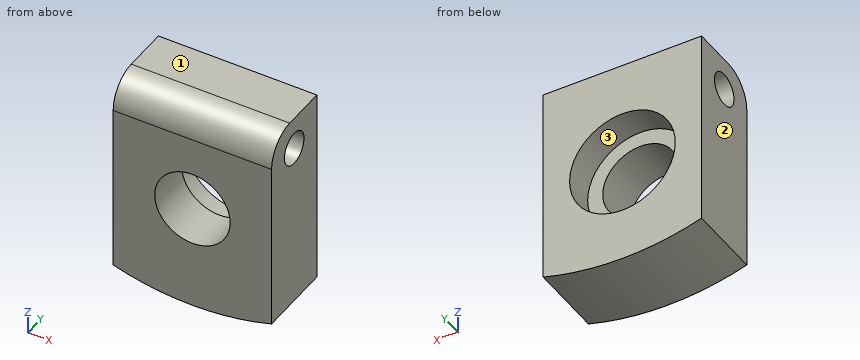
```python
from build123d import *

# Parameters (mm, degrees)
F1_DEPTH       = 30
F3_D           = 30
F3_CBORE_D     = 42
F3_CBORE_DEPTH = 12
F5_R           = 12
F6_D           = 13


with BuildPart() as f1:
    # F0 (on Front) → F1 (new body)
    with BuildSketch(Plane.XZ):
        with BuildLine():
            Line((31.5, 52.105192), (-31.5, 52.105192))
            Line((-31.5, 52.105192), (-31.5, -27.19897))
            ThreePointArc((-31.5, -27.19897), (0, -31.894808), (31.5, -27.19897))
            Line((31.5, -27.19897), (31.5, 52.105192))
        make_face()
    extrude(amount=F1_DEPTH)

    # F3 (through all)
    with Locations(Plane(origin=(0, 0, 0), x_dir=(-1, 0, 0), z_dir=(0, 1, 0))):
        with Locations((0, 10.105192)):
            CounterBoreHole(F3_D / 2, F3_CBORE_D / 2, F3_CBORE_DEPTH)

    # F5
    f5_edges = [f1.edges().sort_by_distance(p)[0] for p in [
        (0, -30, 52.105192),
    ]]
    fillet(f5_edges, radius=F5_R)

    # F6 (through all)
    with Locations(Plane.YZ.offset(31.5)):
        with Locations((-15, 39.105192)):
            Hole(F6_D / 2)


solid = f1.part
```
Check sheet for the modelled part. Datum: model origin and axes. Units: mm. Face numbers are marked on the shaded views. Round coordinates to 2 decimals unless told otherwise and drop trailing zeros. Loops run counter-clockwise (first coordinate to the right, second up) from the corner with the lowest first, then second, coordinate; pieces in that order, holes last. Notation, with made-up numbers: (6.5, 51.25) - (25.5, 51.25) arc R24 ccw to (25.5, 67.25) - close; hole circle Ø5 at (9, 83.25). An arc over 180 degrees is marked (long way). Answer as a JSON object with one key per item and string values. Group by question number.
Q1. Sectioned sample at B-B, the plane x = 0. Enter the section's corners in (y, z), plus the area to 3 significant figures.
Q2. Sectioned sample at D-D, the plane y = -24.25. Enter the section's corners in (x, z).
Q3. Scan lines: line 1 along Z through (x, y) = (0, -7); line 2 along Z through (x, y) = (-7, -12.25); line 3 along Z through (x, y) = (17.5, -9.75). Record each from-to range of solid material in increasing order. Write a range as [from, to].
Q4. Mould release check, pull along Z, two halves, no side actions. Record for the marked faces 1, 2 and 3: released by +Z, released by -Z, zero draft, split by the parting line, or undercut.
Q5. Sectioned sample at C-C, the plane z = -0.5. Enter the section's corners in (x, y).
Q6. Sectioned sample at A-A, the plane y = -15. Enter the section's corners in (x, z), plus the area to 3 significant figures.
Q7. Gauge pin test, flat end, axial feed: P1, Ø8, axis at x = 1, y = -15.5, coming from the -Z side. Record the tip position at first contact, or that the pin passes through.
Solution:
{
 "1": {"outline": "(-30, -31.89) - (0, -31.89) - (0, -10.89) - (-12, -10.89) - (-12, -4.89) - (-30, -4.89) - close; (-30, 25.11) - (-12, 25.11) - (-12, 31.11) - (0, 31.11) - (0, 52.11) - (-18, 52.11) arc R12 ccw to (-30, 40.11) - close; hole circle Ø13 at (-15, 39.11)", "area": "1,310 mm²"},
 "2": {"outline": "(-31.5, -27.2) arc R108 ccw to (31.5, -27.2) - (31.5, 50.35) - (-31.5, 50.35) - close; hole circle Ø30 at (0, 10.11)"},
 "3": {"line 1": "z = [-31.89, -10.89], [31.11, 52.11]", "line 2": "z = [-31.67, -3.16], [23.37, 33.22], [44.99, 52.11]", "line 3": "z = [-30.47, -1.5], [21.71, 35.27], [42.94, 52.11]"},
 "4": {"face 1": "released by +Z", "face 2": "zero draft", "face 3": "undercut"},
 "5": {"outline": "(-31.5, -30) - (-10.61, -30) - (-10.61, -12) - (-18.13, -12) - (-18.13, 0) - (-31.5, 0) - close; (10.61, -30) - (31.5, -30) - (31.5, 0) - (18.13, 0) - (18.13, -12) - (10.61, -12) - close"},
 "6": {"outline": "(-31.5, -27.2) arc R108 ccw to (31.5, -27.2) - (31.5, 32.61) - (-31.5, 32.61) - close; (-31.5, 45.61) - (31.5, 45.61) - (31.5, 52.11) - (-31.5, 52.11) - close; hole circle Ø30 at (0, 10.11)", "area": "3,670 mm²"},
 "7": {"P1": "stops at z = -31.89"}
}
